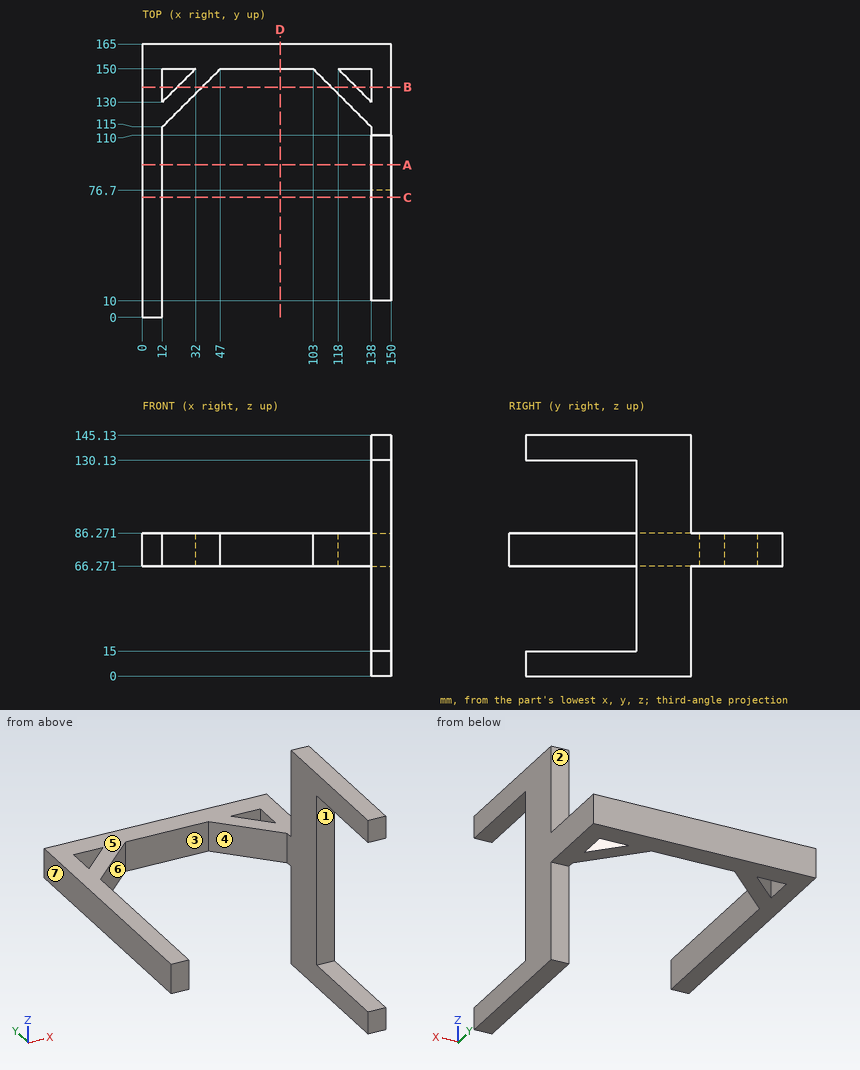
Geometry: see drawing. Coordinates: mm, zero at the bounding-box minimum. A direction names the side the tool comes from. Give positions to 0.01 mm unless a question says otherwise; leave off trailing zeros. Write each loop counter-clockwise with the first axis right and the second up, starting at its lowest first coordinate (ties: lowest second). Pieces come first, ordered by that corner, then holes. Notation, with made-up numbers: M 80,33.5 L 112,33.5 A35 cw 112,69.5 Z; hole C 60.5,31.5 d7. An arc over 180 degrees is marked long. Answer in a Markdown table with one row per item. Add a question column.
(1) Section A-A on y = 92. Return loops of the section in (x, z).
(2) Reachability of the marked faces 1, 2 and 3 from +Z, -Z, +X, -X, +Y, -Y: full face, straight path, thin tool, end or side. Return the list, or none.
(3) Ray query, line 1 (X direction, y = 140, z = 76); line 2 (Y direction, x = 15.5, z = 71); line 3 (Z direction, x = 144.5, y = 22). Return the intervals inside material, ascending.
(4) Section D-D on x = 83. Return loops of the section in (y, z), and give its area (3 significant figures).
(5) First-contact query: pin 1 (9.5 mm diameter, centred on x = 143.5, z = 134.5, fed in from -Y); pin 2 (22 mm diameter, centred on x = 83, z = 78.5, fed in from -Y); pin 3 (6 mm diameter, centred on x = 143.5, z = 78, fed in from -Y); pin 4 (6 mm diameter, centred on x = 134.5, z = 114.5, fed in from -Y). Flat tips, straight axial feed; report the tip coordinate or a pass-through.
(6) Section C-C on y = 72.5. Return loops of the section in (x, z).
(7) Mould query, pull axis X, two halves, no side actions, for the marked faces 4, 5, 6 and 7. Classes: +X half, -X half, draft (parallel to the pull), parting line (faces both ways), or undercut.
(8) Section B-B on y = 139. Return loops of the section in (x, z).
Result set:
| question | item | result |
|---|---|---|
| 1 | outline | M 0,66.27 L 12,66.27 L 12,86.27 L 0,86.27 Z; M 138,0 L 150,0 L 150,145.13 L 138,145.13 Z |
| 2 | face 1 | +X, -Y |
| 2 | face 2 | +Z, +X, -X, +Y |
| 2 | face 3 | +Z, -Z, -Y |
| 3 | line 1 | x = 0 to 12, 22 to 37, 113 to 128, 138 to 150 |
| 3 | line 2 | y = 118.5 to 133.5, 150 to 165 |
| 3 | line 3 | z = 0 to 15, 130.13 to 145.13 |
| 4 | outline | M 150,66.27 L 165,66.27 L 165,86.27 L 150,86.27 Z |
| 4 | area | 300 mm^2 |
| 5 | pin 1 | stops at y = 10 |
| 5 | pin 2 | stops at y = 150 |
| 5 | pin 3 | stops at y = 76.7 |
| 5 | pin 4 | passes through |
| 6 | outline | M 0,66.27 L 12,66.27 L 12,86.27 L 0,86.27 Z; M 138,0 L 150,0 L 150,15 L 138,15 Z; M 138,130.13 L 150,130.13 L 150,145.13 L 138,145.13 Z |
| 7 | face 4 | undercut |
| 7 | face 5 | draft |
| 7 | face 6 | undercut |
| 7 | face 7 | -X half |
| 8 | outline | M 0,66.27 L 12,66.27 L 12,86.27 L 0,86.27 Z; M 21,66.27 L 36,66.27 L 36,86.27 L 21,86.27 Z; M 114,66.27 L 129,66.27 L 129,86.27 L 114,86.27 Z; M 138,66.27 L 150,66.27 L 150,86.27 L 138,86.27 Z |
